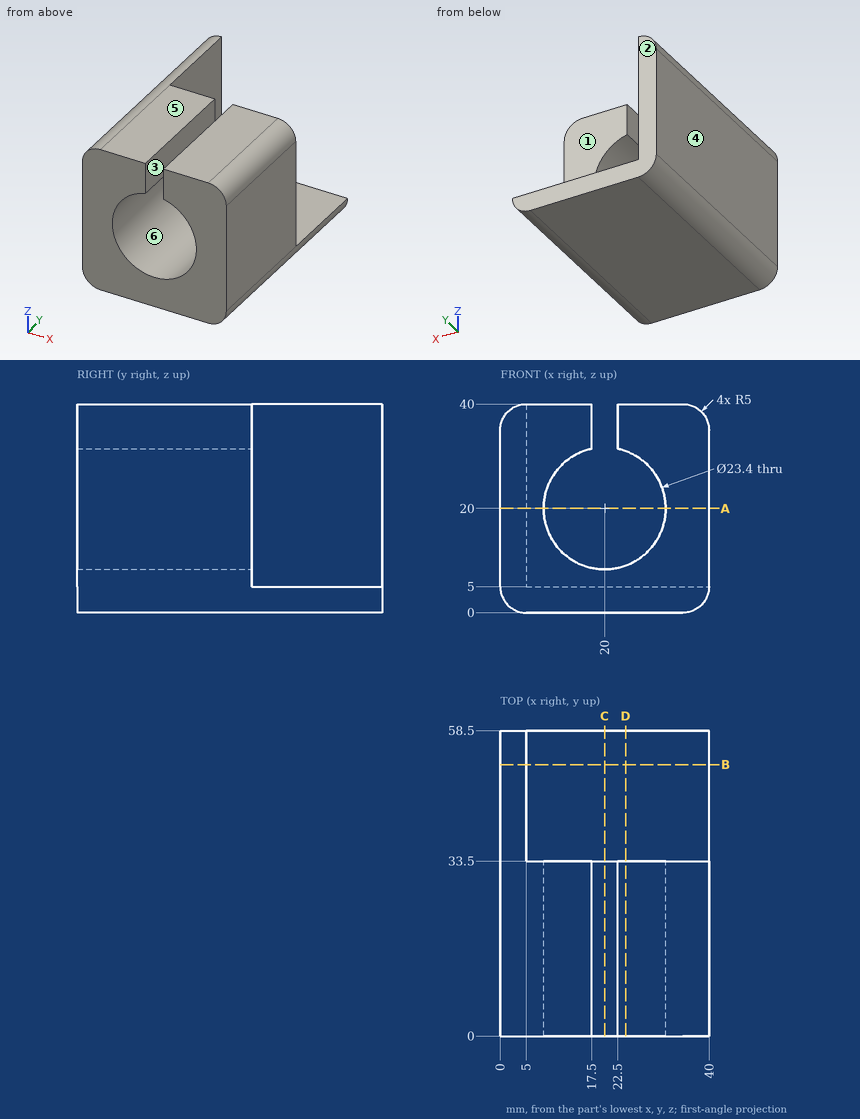
For this review, use the dimensioned drawing (mm, ordinates from the lowest corner) and the shaded views. A direction names the side the tool comes from. Give positions to 0.01 mm unless a question says otherwise; leave off trailing zeros. Order: outer loops, then holes, each group sorted by start corner. A loop starts at its lowest first (then second) coordinate and runs counter-clockwise, first axis right, second up. Notation, with made-up numbers: (20.25, -37.75) -> (79.25, -37.75) arc R13 ccw to (79.25, -14.75) -> close; hole circle Ø7 at (69.25, 78). An arc over 180 degrees is marked (long way). Write item = value, one per line. Start each with the question number.
(1) For L1, parallel to X at y = 16, z = 20; L2, parallel to X at y = 47, z = 20.5, list the stretches that pass through material, from the lowest coordinate up. Write a range as from..to.
(2) Tool access review of the marked faces 1, 2 and 3: name each direction out of +Z, -Z, +X, -X, +Y, -Y from which nothing blocks a thin tool from reaching the whole face with its end or side.
(3) Take a section at B-B (y = 52). Write out the cut boundary in (x, z).
(4) Draft analysis for pull direction Z (two halves, no side actions). For the marked faces 4, 5 and 6, state which applies: +Z half, -Z half, draft (parallel to the pull), parting line (faces both ways), or undercut.
(5) Take a section at D-D (x = 24). Write out the cut boundary in (y, z) (3 decimals), plus the area to 3 significant figures.
(6) Take a section at C-C (x = 20). Write out the cut boundary in (y, z), plus the area to 3 significant figures.
(7) Take a section at A-A (z = 20). Write out the cut boundary in (x, y), plus the area to 3 significant figures.
(8) For pin 1 Ø17.5 at (x, z) = (15.5, 26) entering from +Y; pin 2 Ø12.5 at (y, z) = (44, 25.5) entering from +X; pin 3 Ø4.5 at (y, z) = (12.5, 37.5) entering from -X, all flat-tipped, find the tip position at first contact; note any pin that passes through.
Returned:
q1.L1 = 0..8.3, 31.7..40
q1.L2 = 0..5
q2.face_1 = +Z, +X, +Y
q2.face_2 = +Z, -Z, +X, -X, +Y
q2.face_3 = +Z, +Y, -Y
q3.outline = (0, 5) arc R5 ccw to (5, 0) -> (35, 0) arc R5 ccw to (40, 5) -> (5, 5) -> (5, 40) arc R5 ccw to (0, 35) -> close
q4.face_4 = draft
q4.face_5 = +Z half
q4.face_6 = undercut
q5.outline = (0, 0) -> (58.5, 0) -> (58.5, 5) -> (33.5, 5) -> (33.5, 9.005) -> (0, 9.005) -> close; (0, 30.995) -> (33.5, 30.995) -> (33.5, 40) -> (0, 40) -> close
q5.area = 728 mm²
q6.outline = (0, 0) -> (58.5, 0) -> (58.5, 5) -> (33.5, 5) -> (33.5, 8.3) -> (0, 8.3) -> close
q6.area = 403 mm²
q7.outline = (0, 0) -> (8.3, 0) -> (8.3, 33.5) -> (5, 33.5) -> (5, 58.5) -> (0, 58.5) -> close; (31.7, 0) -> (40, 0) -> (40, 33.5) -> (31.7, 33.5) -> close
q7.area = 681 mm²
q8.pin_1 = 33.5
q8.pin_2 = 5
q8.pin_3 = 0.01
